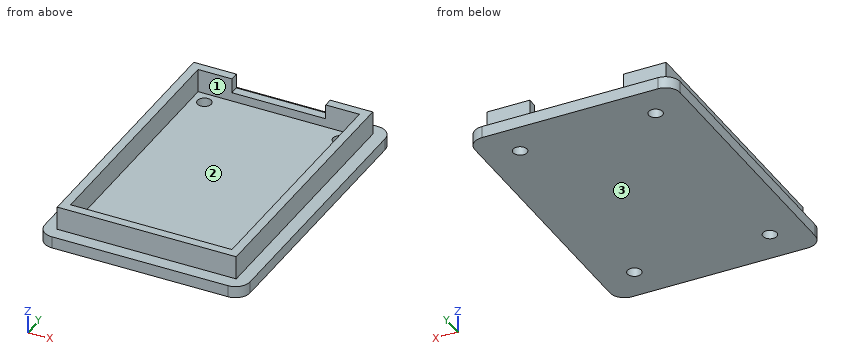
Autodesk Inventor part; units mm, degrees
ref_plane "YZ Plane" through (0, 0, 0) normal (1, 0, 0) x (0, 1, 0)
ref_plane "XZ Plane" through (0, 0, 0) normal (0, 1, 0) x (-1, 0, 0)
ref_plane "XY Plane" through (0, 0, 0) normal (0, 0, 1) x (1, 0, 0)
sketch "Sketch1" plane through (0, 0, 0) normal (0, 0, 1) x (1, 0, 0)
  line L0 (-44.45, 63.5) -> (44.45, 63.5)
  line L1 (44.45, 63.5) -> (44.45, -63.5)
  line L2 (44.45, -63.5) -> (-44.45, -63.5)
  line L3 (-44.45, -63.5) -> (-44.45, 63.5)
  line L4 (0, 63.5) -> (0, -63.5) construction
  point P0 (0, 0)
  point P1 (0, 0)
  dimension "d0" = 88.9
  dimension "d1" = 127
extrude "Extrusion1" add sketch "Sketch1" along normal blind 5.08
fillet "Fillet1" radius 6.35 4 edges at (44.45, 63.5, 2.54) (-44.45, 63.5, 2.54) (44.45, -63.5, 2.54) (-44.45, -63.5, 2.54)
sketch "Sketch2" plane through (0, 0, 5.08) normal (0, 0, 1) x (1, 0, 0)
  line L0 (-38.735, 57.785) -> (38.735, 57.785)
  line L1 (38.735, 57.785) -> (38.735, -57.785)
  line L2 (38.735, -57.785) -> (-38.735, -57.785)
  line L3 (-38.735, -57.785) -> (-38.735, 57.785)
  line L4 (38.1, 63.5) -> (-38.1, 63.5) construction
  line L5 (44.45, -57.15) -> (44.45, 57.15) construction
  line L6 (0, 57.785) -> (0, -57.785) construction
  point P0 (0, 0)
  point P1 (0, 0)
  dimension "d5" = 77.47
  dimension "d6" = 115.57
extrude "Extrusion2" add sketch "Sketch2" along normal blind 10.16
sketch "Sketch3" plane through (0, 0, 15.24) normal (0, 0, 1) x (1, 0, 0)
  line L0 (-34.925, 53.975) -> (34.925, 53.975)
  line L1 (34.925, 53.975) -> (34.925, -53.975)
  line L2 (34.925, -53.975) -> (-34.925, -53.975)
  line L3 (-34.925, -53.975) -> (-34.925, 53.975)
  line L4 (0, -53.975) -> (0, 53.975) construction
  line L5 (38.735, 57.785) -> (-38.735, 57.785)
  line L6 (-38.735, 57.785) -> (-38.735, -57.785)
  point P0 (0, 0)
  point P1 (0, 0)
  dimension "d9" = 3.81
  dimension "d10" = 3.81
extrude "Extrusion3" cut sketch "Sketch3" against normal blind 10.16
sketch "Sketch4" plane through (-38.735, 57.785, 5.08) normal (0, 1, 0) x (1, 0, 0)
  line L0 (77.47, -10.16) -> (0, -10.16)
  line L1 (59.055, -10.16) -> (18.415, -10.16)
  line L2 (18.415, -10.16) -> (18.415, -3.81)
  line L3 (18.415, -3.81) -> (59.055, -3.81)
  line L4 (59.055, -3.81) -> (59.055, -10.16)
  point P0 (38.735, 5.08)
  point P1 (38.735, -10.16)
  dimension "d13" = 40.64
  dimension "d14" = 6.35
extrude "Extrusion4" cut sketch "Sketch4" against normal blind 10.16
sketch "Sketch5" plane through (0, 0, 5.08) normal (0, 0, 1) x (1, 0, 0)
  circle A0 centre (-29.325, 48.375) radius 3
  line L0 (20.32, 53.975) -> (-20.32, 53.975) construction
  line L1 (0, 53.975) -> (0, 7.6098) construction
  line L2 (0, 0) -> (12.3821, 0) construction
  line L3 (-34.925, 53.975) -> (-20.32, 53.975) construction
  line L4 (-34.925, -53.975) -> (-34.925, 53.975) construction
  circle A1 centre (29.325, 48.375) radius 3
  circle A2 centre (-29.325, -48.375) radius 3
  circle A3 centre (29.325, -48.375) radius 3
  dimension "d17" = 6
  dimension "d18" = 5.6
  dimension "d19" = 5.6
extrude "Extrusion5" cut sketch "Sketch5" against normal blind 10
properties part number "EnclosureTop"
Work out the finished part from the listing and answer in its coordinate system (mm). Face numbers are marked on the shaded views. Round coordinates to 2 decimals unless told otherwise and drop trailing zeros. Loops run counter-clockwise (first coordinate to the right, second up) from the corner with the lowest first, then second, coordinate; pieces in that order, holes last. Notation, with made-up numbers: (-26.5, 57) - (27.5, 57) arc R22 cw to (27.5, 69) - close; hole circle Ø3 at (11, 34). An arc over 180 degrees is marked (long way). One line per item, written item: value.
Q1. The mould has two halves that part along X. Classify the marked faces 1, 2 and 3: +X half, -X half, draft (parallel to the pull), parting line (faces both ways), or undercut.
Check values:
face 1: undercut
face 2: undercut
face 3: draft
Q2. Each of these flat-tipped pins is pushed along its axis until it touches: pin 1 Ø5 at (x, z) = (7, 9) entering from -Y (3 decimals); pin 2 Ø2 at (x, y) = (-25.5, -48.5) entering from +Z; pin 3 Ø8 at (y, z) = (19.5, 12) entering from -X (3 decimals). Where does it stop, or does it pass through?
Check values:
pin 1: y = -57.785
pin 2: z = 5.08
pin 3: x = -38.735
Q3. Find section A-A on z = 10.25. Give the vertices of the cut face in (x, y) (3 decimals), and give its area (3 significant figures).
Check values:
outline: (-38.735, -57.785) - (38.735, -57.785) - (38.735, 57.785) - (20.32, 57.785) - (20.32, 53.975) - (34.925, 53.975) - (34.925, -53.975) - (-34.925, -53.975) - (-34.925, 53.975) - (-20.32, 53.975) - (-20.32, 57.785) - (-38.735, 57.785) - close
area: 1,260 mm2
Q4. Straight lines are drawn through the part: probe 1 along Y at (x, z) = (-23, 6) (3 decimals); probe 2 along X at (y, z) = (46, 3.25); probe 3 along X at (y, z) = (-38.5, 14.25) (3 decimals). For each, find the intervals that lie inside material, in ascending order.
Check values:
probe 1: -57.785 to -53.975, 53.975 to 57.785
probe 2: -44.45 to -31.16, -27.49 to 27.49, 31.16 to 44.45
probe 3: -38.735 to -34.925, 34.925 to 38.735
Q5. Find section B-B on y = -39.5. Give the vertices of the cut face in (x, z) (3 decimals).
Check values:
outline: (-44.45, 0) - (44.45, 0) - (44.45, 5.08) - (38.735, 5.08) - (38.735, 15.24) - (34.925, 15.24) - (34.925, 5.08) - (-34.925, 5.08) - (-34.925, 15.24) - (-38.735, 15.24) - (-38.735, 5.08) - (-44.45, 5.08) - close
